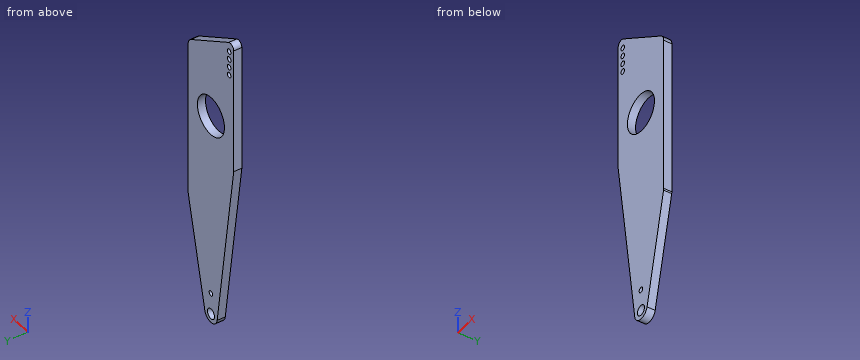
```python
from build123d import *

# Parameters (mm, degrees)
SKETCH1_R           = 3.96875
SKETCH1_R_2         = 15.08125
SKETCH1_R_3         = 2
BOSS_EXTRUDE1_DEPTH = 6.35


with BuildPart() as part:
    # Sketch1 → Boss-Extrude1 (new body)
    with BuildSketch(Plane(origin=(0, 0, 0), x_dir=(1, 0, 0), z_dir=(0, 1, 0))):
        with BuildLine():
            Line((25.4, -82.735721877), (25.4, -202.708825791))
            ThreePointArc((25.4, -202.708825791), (24.549261314, -205.883825791), (22.225, -208.208087105))
            Line((22.225, -208.208087105), (-19.685, -232.404836886))
            ThreePointArc((-19.685, -232.404836886), (-23.495, -232.404836886), (-25.4, -229.105280098))
            Line((-25.4, -229.105280098), (-25.4, -131.278691098))
            Line((-25.4, -131.278691098), (-6.917767735, 0.966806375))
            ThreePointArc((-6.917767735, 0.966806375), (-0.279220673, 6.97941694), (6.818426198, 1.51634072))
            Line((6.818426198, 1.51634072), (25.248569271, -81.357230313))
            ThreePointArc((25.248569271, -81.357230313), (25.362028789, -82.042329806), (25.4, -82.735721877))
        make_face()
        with Locations(Location((0, 0, 0), (0, 0, 270))):
            Circle(SKETCH1_R, mode=Mode.SUBTRACT)
        with Locations(Location((0, -160.246508934, 0), (0, 0, 270))):
            Circle(SKETCH1_R_2, mode=Mode.SUBTRACT)
        with Locations(Location((-20.32, -225.425, 0), (0, 0, 270))):
            Circle(SKETCH1_R_3, mode=Mode.SUBTRACT)
        with Locations(Location((-20.32, -219.075, 0), (0, 0, 270))):
            Circle(SKETCH1_R_3, mode=Mode.SUBTRACT)
        with Locations(Location((-20.32, -212.725, 0), (0, 0, 270))):
            Circle(SKETCH1_R_3, mode=Mode.SUBTRACT)
        with Locations(Location((-20.32, -206.375, 0), (0, 0, 270))):
            Circle(SKETCH1_R_3, mode=Mode.SUBTRACT)
        with Locations(Location((0, -16.51, 0), (0, 0, 270))):
            Circle(SKETCH1_R_3, mode=Mode.SUBTRACT)
    extrude(amount=-BOSS_EXTRUDE1_DEPTH)


solid = part.part
```
CAD build for the part. Positions are in the model's coordinates, mm. Round coordinates to 2 decimals unless told otherwise and drop trailing zeros. Write each loop counter-clockwise with the first axis right and the second up, starting at its lowest first coordinate (ties: lowest second). Pieces come first, ordered by that corner, then holes. Notation, with made-up numbers: (-25.5, 46.5) - (1.5, 46.5) arc R7 cw to (1.5, 59.5) - close; hole circle Ø2 at (23, 5.25). An arc over 180 degrees is marked (long way). Write item = value, one per line. Start each with the question number.
Q1. Band-saw the part on B-B (y = -1.5). Count the separate pieces of the cut face and the enclosed holes in it, then the cut area to 3 significant figures.
Q2. Band-saw the part on C-C (x = 11). Give the cut face in (y, z), then the cut area to 3 significant figures.
Q3. Band-saw the part on A-A (x = 0). Give the cut face in (y, z) (3 decimals).
Q4. Drop flat-ended pins along their axis: pin 1 (1.5 mm diameter, centred on x = 12, y = -4.5, fed in from +Z); pin 2 (3.5 mm diameter, centred on x = -20.32, z = 225.425, fed in from +Y); pin 3 (1 mm diameter, centred on x = 17, y = -1.5, fed in from +Z); pin 4 (3 mm diameter, centred on x = -7.5, y = -5.5, fed in from -Z). Give the stop position or say it passes through.
Q5. Probe L1, parallel to Z at x = 3, y = -4.25; L2, parallel to X at y = -1.25, z = 153; L3, parallel to X at y = -2.5, z = 150. List the from-to ranges inside material, lowest first. Write a range as from..to.
Q6. Band-saw the part on D-D (z = 16.51). Give the cut face in (x, y), then the cut area to 3 significant figures.
Answers below:
q1.separate_pieces = 1
q1.enclosed_holes = 7
q1.area = 8,510 mm2
q2.outline = (-6.35, 17.29) - (0, 17.29) - (0, 149.93) - (-6.35, 149.93) - close; (-6.35, 170.56) - (0, 170.56) - (0, 214.69) - (-6.35, 214.69) - close
q2.area = 1,120 mm2
q3.outline = (-6.35, -6.985) - (0, -6.985) - (0, -3.969) - (-6.35, -3.969) - close; (-6.35, 3.969) - (0, 3.969) - (0, 14.51) - (-6.35, 14.51) - close; (-6.35, 18.51) - (0, 18.51) - (0, 145.165) - (-6.35, 145.165) - close; (-6.35, 175.328) - (0, 175.328) - (0, 221.04) - (-6.35, 221.04) - close
q4.pin_1 = 214.54
q4.pin_2 = through
q4.pin_3 = 211.51
q4.pin_4 = -3.58
q5.L1 = -6.31..-2.6, 2.6..145.47, 175.03..219.31
q5.L2 = -25.4..-13.23, 13.23..25.4
q5.L3 = -25.4..-11.07, 11.07..25.4
q6.outline = (-9.36, -6.35) - (-2, -6.35) - (-2, 0) - (-9.36, 0) - close; (2, -6.35) - (10.83, -6.35) - (10.83, 0) - (2, 0) - close
q6.area = 103 mm2
